The listing builds one solid part. Answer for the finished solid, in the listing's coordinates (mm). A direction names the side the tool comes from. Coordinates: 2 decimals unless noted, no trailing zeros. Order: outer loops, then holes, each group sorted by start corner. A loop starts at its lowest first (then second) coordinate and runs counter-clockwise, first axis right, second up. Notation, with made-up numbers: (-38, -29.5) -> (11, -29.5) arc R20 cw to (11, -4.5) -> close; hole circle Ø6 at (34, -34.5). An arc over 180 degrees is marked (long way). Return JSON: item names as keys, results as strings.
Autodesk Inventor part; units mm, degrees
ref_plane "YZ Plane" through (0, 0, 0) normal (1, 0, 0) x (0, 1, 0)
ref_plane "XZ Plane" through (0, 0, 0) normal (0, 1, 0) x (-1, 0, 0)
ref_plane "XY Plane" through (0, 0, 0) normal (0, 0, 1) x (1, 0, 0)
sketch "Sketch1" plane through (0, 0, 0) normal (0, 1, 0) x (-1, 0, 0)
  line L0 (7.5, -7.5) -> (-7.5, -7.5)
  line L1 (-7.5, -7.5) -> (-7.5, 7.5)
  line L2 (-7.5, 7.5) -> (7.5, 7.5)
  line L3 (7.5, 7.5) -> (7.5, -7.5)
  line L4 (7.5, -7.5) -> (-7.5, 7.5) construction
  line L5 (-7.5, -7.5) -> (7.5, 7.5) construction
  point P0 (0, 0)
  dimension "d0" = 15
  dimension "d1" = 15
extrude "Extrusion1" add sketch "Sketch1" along normal blind 0.6
sketch "Sketch2" plane through (0, 0.6, 0) normal (0, 1, 0) x (1, 0, 0)
  circle A0 centre (0, 0) radius 7.125
  circle A1 centre (0, 0) radius 7.5
  dimension "d4" = 14.25
  dimension "d5" = 15
extrude "Extrusion2" add sketch "Sketch2" along normal blind 0.6
equation "\"d1\" = d0"
properties part number "dot_antirol"
Item 1: The part is cut by section A-A on z = 2. Determine the outline of the cut face in (x, y).
Answer list:
{"outline": "(-7.5, 0) -> (7.5, 0) -> (7.5, 0.6) -> (7.23, 0.6) -> (7.23, 1.2) -> (6.84, 1.2) -> (6.84, 0.6) -> (-6.84, 0.6) -> (-6.84, 1.2) -> (-7.23, 1.2) -> (-7.23, 0.6) -> (-7.5, 0.6) -> close"}
Item 2: Find the intervals of material crossed by probe 1 along Z at (x, y) = (0, 0.95) (3 decimals); probe 2 along Y at (x, z) = (-6.5, 5.25), in increasing order.
Answer list:
{"probe 1": "-7.5 to -7.125, 7.125 to 7.5", "probe 2": "0 to 0.6"}
Item 3: Which of the six approach directions +Z, -Z, +X, -X, +Y, -Y give full straight-line access (tool end or side, diameter ignored) to faces 1 (the flat face through (-6, 0.6, 6)), 2 (the flat face through (-6, 0.6, -6)), 3 (the flat face through (6, 0.6, 6)), 4 (the flat face through (0, 0.6, 0)), 5 (the flat face through (6, 0.6, -6))?
Answer list:
{"face 1": "+Z, -X, +Y", "face 2": "-Z, -X, +Y", "face 3": "+Z, +X, +Y", "face 4": "+Y", "face 5": "-Z, +X, +Y"}
Item 4: The part is cut by section B-B on x = -6.25. Determine the outline of the cut face in (y, z).
Answer list:
{"outline": "(0, -7.5) -> (0.6, -7.5) -> (0.6, -4.15) -> (1.2, -4.15) -> (1.2, -3.42) -> (0.6, -3.42) -> (0.6, 3.42) -> (1.2, 3.42) -> (1.2, 4.15) -> (0.6, 4.15) -> (0.6, 7.5) -> (0, 7.5) -> close"}
Item 5: The part is cut by section C-C on y = 0.85. Determine the outline of the cut face in (x, z) (3 decimals).
Answer list:
{"outline": "circle Ø15 at (0, 0); hole circle Ø14.25 at (0, 0)"}
